from build123d import *

# Parameters (mm, degrees)
F0_R         = 2.1251138046
F1_DEPTH     = 5
F0_W         = 14.2144468555
F0_H         = 18.6405025888
F2_DEPTH     = 130
F3_W         = 14.2144468555
F3_H         = 3
F4_DEPTH     = 10.03026
F5_R         = 5
F6_R         = 3
F7_T1_DEPTH  = 4.2144468555
F7_T6_DEPTH  = 13.6405025888
F7_S7_R      = 2.1251138046
F7_T8_DEPTH  = 9
F7_T10_ANGLE = 90
F7_T12_ANGLE = 90
F7_T16_DEPTH = 13.6405025888
F7_S17_R     = 2.1251138046
F7_T18_DEPTH = 9


# Not quite as in the source:
# - a fillet or chamfer that OpenCascade refuses, or shapes differently, is made with other operations: its cross-section is extruded or revolved along the edge and cut away or added


with BuildPart() as f1:
    # F0 (on Front) → F1 (new body)
    with BuildSketch(Plane.XZ):
        Polygon((16.5932904929, 31.273946166), (-29.8148933798, 31.273946166), (-29.8148933798, -17.4539741129), (-13.7278847396, -17.4539741129), (-13.7278847396, 1.186528476), (0.4865621158, 1.186528476), (0.4865621158, -17.4539741129), (16.5932904929, -17.4539741129), align=None)
        with Locations((-19.3455703557, -7.9430211366)):
            Circle(F0_R, mode=Mode.SUBTRACT)
        with Locations((5.1544296443, -7.9430211366)):
            Circle(F0_R, mode=Mode.SUBTRACT)
        with Locations((-19.3455703557, 22.9763388634)):
            Circle(F0_R, mode=Mode.SUBTRACT)
        with Locations((5.1544296443, 22.9763388634)):
            Circle(F0_R, mode=Mode.SUBTRACT)
    extrude(amount=F1_DEPTH)

    # F0 (on Front) → F2 (join)
    with BuildSketch(Plane.XZ):
        with Locations((-6.6206613119, -8.1337228185)):
            Rectangle(F0_W, F0_H)
    extrude(amount=F2_DEPTH)

    # F3 (on face) → F4 (join)
    with BuildSketch(Plane.XY.offset(1.186528476)):
        with Locations((-6.6206613119, -128.5)):
            Rectangle(F3_W, F3_H)
    extrude(amount=F4_DEPTH)

    # F5
    f5_edges = [f1.edges().sort_by_distance(p)[0] for p in [
        (0.486562, -66, 1.186528),
        (-13.727885, -66, 1.186528),
        (-13.727885, -128.5, 11.216788),
        (0.486562, -128.5, 11.216788),
    ]]
    fillet(f5_edges, radius=F5_R)

    # F6
    f6_edges = [f1.edges().sort_by_distance(p)[0] for p in [
        (-29.814893, -2.5, 31.273946),
        (16.59329, -2.5, 31.273946),
        (-29.814893, -2.5, -17.453974),
        (16.59329, -2.5, -17.453974),
    ]]
    fillet(f6_edges, radius=F6_R)

    # F7: chamfer of 4 on 2 edges, made by hand

    # F7_s2 → F7_t1 (join)
    with BuildSketch(Plane.YZ.offset(-8.7278847396)):
        Polygon((-5, 5.186528476), (-9, 1.186528476), (-5, 1.186528476), align=None)
    extrude(amount=F7_T1_DEPTH)


with BuildPart() as f7_tool4:
    # F7_s5 → F7_t6 (new body)
    with BuildSketch(Plane.XY.offset(-3.813471524)):
        Polygon((4.4865621158, -5), (0.4865621158, -9), (0.4865621158, -5), align=None)
    extrude(amount=-F7_T6_DEPTH)

    # F7_s7 → F7_t8 (cut, symmetric)
    with BuildSketch(Plane.XZ.offset(7)):
        with Locations((5.1544296443, -7.9430211366)):
            Circle(F7_S7_R)
    extrude(amount=F7_T8_DEPTH, both=True, mode=Mode.SUBTRACT)


with BuildPart() as f1_1:
    add(f1.part)

    # F7_t3: union F7_tool4
    add(f7_tool4.part)

    # F7_s9 → F7_t10 (revolve)
    with BuildSketch(Plane.XY.offset(-3.813471524)):
        Polygon((4.4865621158, -5), (0.4865621158, -9), (0.4865621158, -5), align=None)
    revolve(axis=Axis((-4.5134378842, -5, -3.813471524), (0, -1, 0)), revolution_arc=F7_T10_ANGLE)

    # F7_s11 → F7_t12 (revolve)
    with BuildSketch(Plane.YZ.offset(-8.7278847396)):
        Polygon((-5, 5.186528476), (-9, 1.186528476), (-5, 1.186528476), align=None)
    revolve(axis=Axis((-8.7278847396, -5, -3.813471524), (0, -1, 0)), revolution_arc=F7_T12_ANGLE)


with BuildPart() as f7_tool14:
    # F7_s15 → F7_t16 (new body)
    with BuildSketch(Plane.XY.offset(-17.4539741129)):
        Polygon((-17.7278847396, -5), (-13.7278847396, -9), (-13.7278847396, -5), align=None)
    extrude(amount=F7_T16_DEPTH)

    # F7_s17 → F7_t18 (cut, symmetric)
    with BuildSketch(Plane.XZ.offset(7)):
        with Locations((-19.3455703557, -7.9430211366)):
            Circle(F7_S17_R)
    extrude(amount=F7_T18_DEPTH, both=True, mode=Mode.SUBTRACT)


with BuildPart() as f1_2:
    add(f1_1.part)

    # F7_t13: union F7_tool14
    add(f7_tool14.part)


solid = f1_2.part
Could you check a few things on this model? Use its own coordinates, in mm. A direction names the side the tool comes from. Coordinates: 2 decimals unless noted, no trailing zeros. Order: outer loops, then holes, each group sorted by start corner. A loop starts at its lowest first (then second) coordinate and runs counter-clockwise, first axis right, second up. Notation, with made-up numbers: (26, -19.75) -> (42, -19.75) arc R16 ccw to (42, -6.75) -> close; hole circle Ø8 at (59.25, 49.25). An arc over 180 degrees is marked (long way). One line per item, written item: value. Start each with the question number.
1) We'd pull the mould along Z, two halves only. Please class faces 6 (the conical face through (-13.293, -7.472, 0.853)), 7 (the cylindrical face through (4.878, -2.465, 25.083)), 8 (the flat face through (0.487, -70, -11)): +Z half, -Z half, draft (parallel to the pull), parting line (faces both ways), or undercut.
2) I'm going to push flat-ended pins straight in: pin 1 (5.5 mm diameter, centred on x = 5.15, z = -7.94, fed in from -Y); pin 2 (10 mm diameter, centred on x = 6.5, y = -70.5, fed in from +Z); pin 3 (5.5 mm diameter, centred on x = -19.35, z = 22.98, fed in from -Y); pin 4 (4.5 mm diameter, centred on x = -7, y = -48, fed in from +Z). Where does each tip first touch, or does it pass through?
3) Imagine slicing it at B-B on y = -38. List the corners of the cut face in (x, z) for me.
4) Imagine slicing it at C-C on x = 11. List the corners of the cut face in (y, z) for me, plus the area to 3 significant figures.
5) Which directions (+Z, -Z, +X, -X, +Y, -Y) give clear straight access to the entire face, cutting with the end or side of a thin tool? Please do faces 1 (the flat face through (-7, -128, 11.217)), 2 (the flat face through (-6.65, -6.972, 3.215)), 3 (the cylindrical face through (-12, -128, 10)), 4 (the cylindrical face through (-0.939, -68.826, -0.317)), 5 (the cylindrical face through (-0.939, -128.479, 9.713)).
6) If I drill on L1, parallel to Y at x = -12, z = 9.5; L2, parallel to Z at x = -8, y = -98; L3, parallel to Y at x = -23, z = 2.5, over which ranges is the centre line in solid material (lowest first)? Write a range as [from, to].
7) Imagine slicing it at A-A on x = -19. List the corners of the cut face in (y, z) for me.
Answer list:
1. face 6: +Z half
1. face 7: undercut
1. face 8: draft
2. pin 1: stops at y = -7.09
2. pin 2: passes through
2. pin 3: stops at y = -5
2. pin 4: stops at z = 1.19
3. outline: (-13.73, -17.45) -> (0.49, -17.45) -> (0.49, -3.81) arc R5 ccw to (-4.51, 1.19) -> (-8.73, 1.19) arc R5 ccw to (-13.73, -3.81) -> close
4. outline: (-5, -17.45) -> (0, -17.45) -> (0, 31.27) -> (-5, 31.27) -> close
4. area: 244 mm2
5. face 1: +Z, +X, -X, -Y
5. face 2: +Z, +X, -X
5. face 3: +Z, -X, -Y
5. face 4: +Z, +X
5. face 5: +Z, +X, -Y
6. L1: y = [-130, -127], [-5, 0]
6. L2: z = [-17.45, 1.19]
6. L3: y = [-5, 0]
7. outline: (-5, -17.45) -> (0, -17.45) -> (0, -10.04) -> (-5, -10.04) -> close; (-5, -5.85) -> (0, -5.85) -> (0, 20.88) -> (-5, 20.88) -> close; (-5, 25.07) -> (0, 25.07) -> (0, 31.27) -> (-5, 31.27) -> close
